Can you work these out from the model? Positions are in its coordinate system, mm. Face numbers are marked on the shaded views. A direction names the side the tool comes from. Round coordinates to 2 decimals unless told otherwise and drop trailing zeros. Order: outer loops, then holes, each group sorted by start corner. A loop starts at its lowest first (then second) coordinate and runs counter-clockwise, first axis right, second up.
Q1. If we section it at B-B (y = 17.5): Please give me the cut outline in (x, z) (3 decimals), plus the area to 3 significant figures.
Q2. If I drill on line 1 (X direction, y = 7.5, z = -74.5) (3 decimals); line 2 (Z direction, x = 104, y = -8.5) (3 decimals); line 3 (X direction, y = -27, z = -27.5), over which ranges is the centre line in solid material (lowest first)?
Q3. Will these pins go through, and if not, where does the flat tip stop? P1, Ø1.6, axis at x = 78, z = -129, coming from the -Y side (3 decimals); P2, Ø2.5, axis at x = -1.5, z = -87, coming from the -Y side; P3, Ø12, axis at x = 108.5, z = -27, coming from the +Y side.
Q4. If we section it at D-D (x = 107.5): Please give me the cut outline in (y, z) (3 decimals), plus the area to 3 significant figures.
Q5. We'd pull the mould along X, two halves only. Please class the marked faces 1, 2 and 3: pulls with the +X half, pulls with the -X half, needs draft (parallel to the pull), parting line crosses it, or undercut.
Q6. If we section it at C-C (z = -32.5): Please give me the cut outline in (x, y) (3 decimals).
Q7. If we section it at A-A (x = 31): Please give me the cut outline in (y, z) (3 decimals), plus the area to 3 significant figures.
Q8. For the marked faces 4, 5 and 6, which set-ups out of +Z, -Z, +X, -X, +Y, -Y let a thin tool reach every point of the face, with its end or its side?
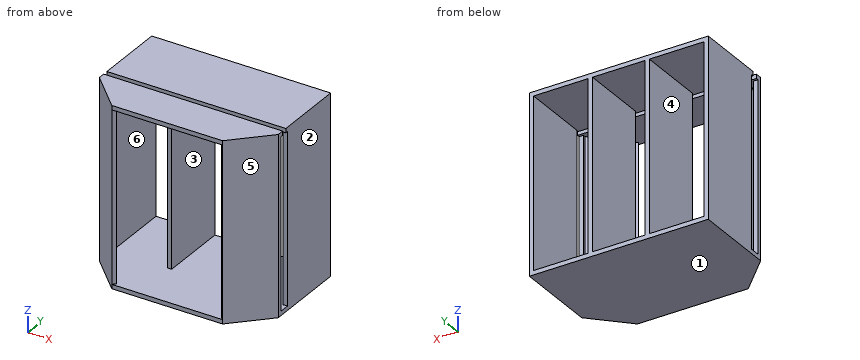
Autodesk Inventor part; units mm, degrees
ref_plane "YZ Plane" through (0, 0, 0) normal (1, 0, 0) x (0, 1, 0)
ref_plane "XZ Plane" through (0, 0, 0) normal (0, 1, 0) x (-1, 0, 0)
ref_plane "XY Plane" through (0, 0, 0) normal (0, 0, 1) x (1, 0, 0)
sketch "Sketch2" plane through (0, 0, 0) normal (0, 1, 0) x (-1, 0, 0)
  line L0 (0, 0) -> (-127, 0)
  line L1 (-127, 0) -> (-127, -127)
  line L2 (-127, -127) -> (0, -127)
  line L3 (0, -127) -> (0, 0)
  line L4 (0, 0) -> (-40.7416, 0)
  line L5 (-40.7416, 0) -> (-40.7416, -127)
  line L6 (-40.7416, -127) -> (0, -127)
  line L7 (0, -127) -> (0, 0)
  line L8 (3.175, 3.175) -> (-130.175, 3.175)
  line L9 (-130.175, 3.175) -> (-130.175, -130.175)
  line L10 (-130.175, -130.175) -> (3.175, -130.175)
  line L11 (3.175, -130.175) -> (3.175, 3.175)
  line L12 (-127, 0) -> (-86.2584, 0)
  line L13 (-86.2584, 0) -> (-86.2584, -127)
  line L14 (-86.2584, -127) -> (-127, -127)
  line L15 (-127, -127) -> (-127, 0)
  line L16 (-40.7416, -44.9087) -> (-43.9166, -44.9087) construction
  line L17 (-86.2584, -51.4533) -> (-83.0834, -51.4533) construction
  line L18 (-43.9166, 0) -> (-83.0834, 0)
  line L19 (-83.0834, 0) -> (-83.0834, -127)
  line L20 (-83.0834, -127) -> (-43.9166, -127)
  line L21 (-43.9166, -127) -> (-43.9166, 0)
  dimension "d11" = 127
  dimension "d12" = 127
  dimension "d13" = 40.7416
  dimension "d14" = 3.175
  dimension "d15" = 40.7416
  dimension "d16" = 3.175
  dimension "d17" = 3.175
extrude "Extrusion2" add sketch "Sketch2" along normal blind 50.8 contours L5 L2 L21 L0 | L19 L2 L13 L0 | L11 L10 L9 L8
sketch "Sketch3" plane through (0, 0, 0) normal (0, -1, 0) x (1, 0, 0)
  line L0 (130.175, 3.175) -> (130.175, -130.175)
  line L1 (-3.175, -130.175) -> (-3.175, 3.175)
  line L2 (130.175, 3.175) -> (-3.175, 3.175)
  line L3 (-3.175, 3.175) -> (-3.175, 0)
  line L4 (-3.175, 0) -> (130.175, 0)
  line L5 (130.175, 0) -> (130.175, 3.175)
  line L6 (130.175, -130.175) -> (-3.175, -130.175)
  line L7 (-3.175, -130.175) -> (-3.175, -127)
  line L8 (-3.175, -127) -> (130.175, -127)
  line L9 (130.175, -127) -> (130.175, -130.175)
  point P0 (0, 0)
  dimension "d20" = 133.35
  dimension "d21" = 3.175
extrude "Extrusion3" add sketch "Sketch3" along normal blind 1.905 contours L0 L4 L1 L2
sketch "Sketch4" plane through (0, 0, 0) normal (0, -1, 0) x (1, 0, 0)
  line L0 (130.175, 0) -> (130.175, -130.175)
  line L1 (130.175, -130.175) -> (-3.175, -130.175)
  line L2 (-3.175, -130.175) -> (-3.175, -127)
  line L3 (-3.175, -127) -> (130.175, -127)
  line L4 (130.175, -127) -> (130.175, -130.175)
  point P0 (0, 0)
  dimension "d24" = 133.35
  dimension "d25" = 3.175
extrude "Extrusion4" add sketch "Sketch4" along normal blind 7.62
sketch "Sketch5" plane through (0, -7.62, 0) normal (0, -1, 0) x (1, 0, 0)
  line L0 (130.175, -130.175) -> (-3.175, -130.175)
  line L1 (130.175, -130.175) -> (-3.175, -130.175)
  line L2 (-3.175, -130.175) -> (-3.175, 3.175)
  line L3 (-3.175, 3.175) -> (130.175, 3.175)
  line L4 (130.175, 3.175) -> (130.175, -130.175)
  line L5 (127, 0) -> (0, 0)
  line L6 (0, 0) -> (0, -127)
  line L7 (0, -127) -> (127, -127)
  line L8 (127, -127) -> (127, 0)
  point P0 (0, 0)
  dimension "d32" = 3.175
extrude "Extrusion5" add sketch "Sketch5" along normal blind 3.175
sketch "Sketch6" plane through (0, -10.795, 0) normal (0, -1, 0) x (1, 0, 0)
  line L0 (130.175, -127) -> (130.175, 3.175)
  line L1 (-3.175, -130.175) -> (-3.175, 3.175)
  line L2 (130.175, 3.175) -> (-3.175, 3.175)
  line L3 (-3.175, 3.175) -> (-3.175, 0)
  line L4 (-3.175, 0) -> (130.175, 0)
  line L5 (130.175, 0) -> (130.175, 3.175)
  point P0 (0, 0)
extrude "Extrusion6" add sketch "Sketch6" against normal blind 5.08
sketch "Sketch7" plane through (-3.175, -10.795, 3.175) normal (0, 0, 1) x (1, 0, 0)
  line L0 (0, 0) -> (133.35, 0) construction
  line L1 (0, 0) -> (0, -25.4) construction
  line L2 (0, -25.4) -> (25.4, -25.4) construction
  line L3 (133.35, 0) -> (133.35, -25.4) construction
  line L4 (133.35, -25.4) -> (107.95, -25.4) construction
  line L5 (0, 0) -> (25.4, -25.4)
  line L6 (25.4, -25.4) -> (107.95, -25.4)
  line L7 (107.95, -25.4) -> (133.35, 0)
  line L8 (0, 0) -> (133.35, 0)
  point P0 (3.175, 10.795)
  dimension "d33" = 25.4
  dimension "d34" = 25.4
  dimension "d35" = 25.4
  dimension "d36" = 25.4
extrude "Extrusion7" add sketch "Sketch7" against normal blind 3.175
sketch "Sketch8" plane through (130.175, 50.8, -130.175) normal (0, 0, -1) x (-1, 0, 0)
  line L0 (107.95, -86.995) -> (133.35, -61.595)
  line L1 (133.35, -61.595) -> (107.95, -86.995)
  line L2 (25.4, -86.995) -> (107.95, -86.995)
  line L3 (107.95, -86.995) -> (25.4, -86.995)
  line L4 (0, -56.515) -> (0, -61.595)
  line L5 (25.4, -86.995) -> (0, -61.595)
  line L6 (0, -61.595) -> (133.35, -61.595)
  point P0 (130.175, -50.8)
extrude "Extrusion8" add sketch "Sketch8" against normal blind 3.175
sketch "Sketch9" plane through (22.225, -36.195, -127) normal (-0.7071068, -0.7071068, 0) x (-0.7071068, 0.7071068, 0)
  line L0 (35.921, 0) -> (35.921, 3.175)
  line L1 (39.5131, -130.175) -> (-54.7796, -130.175)
  line L2 (35.921, 3.175) -> (-0.0076, 3.175)
  line L3 (-0.0076, 3.175) -> (-0.0076, -130.175)
  line L4 (-0.0076, -130.175) -> (35.921, -130.175)
  line L5 (35.921, -130.175) -> (35.921, 3.175)
  point P0 (41.3092, -127)
  point P1 (35.921, -130.175)
  point P2 (35.921, 0)
extrude "Extrusion9" add sketch "Sketch9" against normal blind 3.175
sketch "Sketch10" plane through (104.775, -36.195, 3.175) normal (0.7071068, -0.7071068, 0) x (-0.7071068, -0.7071068, 0)
  line L0 (0, 0) -> (0, 3.175)
  line L1 (-35.921, 133.35) -> (0, 133.35)
  line L2 (0, 0) -> (-35.921, 0)
  line L3 (-35.921, 0) -> (-35.921, 133.35)
  line L4 (-35.921, 133.35) -> (0, 133.35)
  line L5 (0, 133.35) -> (0, 0)
  point P0 (48.4934, 3.175)
extrude "Extrusion10" add sketch "Sketch10" against normal blind 3.175
properties part number "BeadCompartments_4"
Solution:
1. outline: (-3.175, -130.175) - (130.175, -130.175) - (130.175, 3.175) - (-3.175, 3.175) - close; hole (0, -127) - (40.742, -127) - (40.742, 0) - (0, 0) - close; hole (43.917, -127) - (83.083, -127) - (83.083, 0) - (43.917, 0) - close; hole (86.258, -127) - (127, -127) - (127, 0) - (86.258, 0) - close
1. area: 2,460 mm2
2. line 1: x = -3.175 to 0, 40.742 to 43.917, 83.083 to 86.258, 127 to 130.175
2. line 2: z = -130.175 to -127, 0 to 3.175
2. line 3: x = 13.03 to 17.52, 109.48 to 113.97
3. P1: stops at y = -36.195
3. P2: stops at y = -13.72
3. P3: stops at y = -21.98
4. outline: (-33.47, -130.175) - (50.8, -130.175) - (50.8, -127) - (-28.98, -127) - (-28.98, 0) - (-5.715, 0) - (-5.715, 3.175) - (-33.47, 3.175) - close; (-1.905, 0) - (50.8, 0) - (50.8, 3.175) - (-1.905, 3.175) - close
4. area: 1,090 mm2
5. face 1: needs draft
5. face 2: pulls with the +X half
5. face 3: undercut
6. outline: (-3.175, -10.795) - (22.23, -36.2) - (24.475, -33.955) - (0, -9.48) - (0, -7.62) - (-3.175, -7.62) - close; (-3.175, 0) - (0, 0) - (0, 50.8) - (-3.175, 50.8) - close; (40.742, 0) - (43.917, 0) - (43.917, 50.8) - (40.742, 50.8) - close; (83.083, 0) - (86.258, 0) - (86.258, 50.8) - (83.083, 50.8) - close; (102.53, -33.95) - (104.775, -36.195) - (130.175, -10.795) - (130.175, -7.62) - (127, -7.62) - (127, -9.48) - close; (127, 0) - (130.175, 0) - (130.175, 50.8) - (127, 50.8) - close
7. outline: (-36.195, -130.175) - (50.8, -130.175) - (50.8, -127) - (-36.195, -127) - close; (-36.195, 0) - (-5.715, 0) - (-5.715, 3.175) - (-36.195, 3.175) - close; (-1.905, 0) - (50.8, 0) - (50.8, 3.175) - (-1.905, 3.175) - close
7. area: 540 mm2
8. face 4: +Y, -Y
8. face 5: +Z, -Z, +X, -Y
8. face 6: +Y
